Can you work these out from the model? Positions are in its coordinate system, mm. Face numbers are marked on the shaded views. A direction names the side the tool comes from. Give positions to 0.01 mm unless a question says otherwise; leave off trailing zeros. Order: outer loops, then holes, each group sorted by start corner. A loop starts at its lowest first (then second) coordinate and runs counter-clockwise, first axis right, second up. Notation, with made-up numbers: (-38, 87) - (8, 87) arc R32 ccw to (8, 123) - close; hole circle Ø8 at (58.25, 65). An arc over 180 degrees is marked (long way). One line per question, with ' | ' between items.
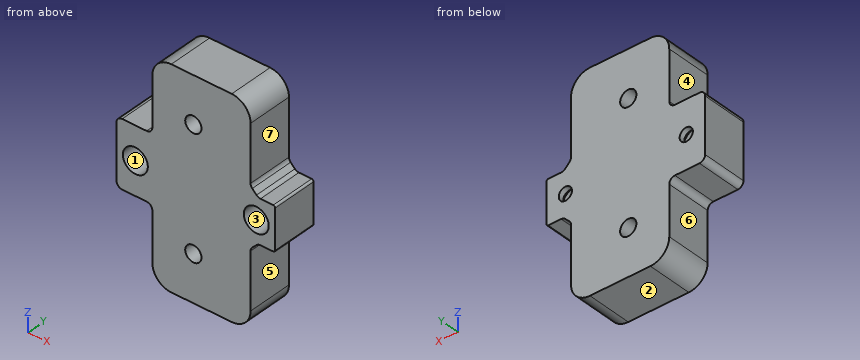
Autodesk Fusion 360 part; units mm, degrees
sketch "Sketch1" plane through (0, 0, 0) normal (0, 1, 0) x (1, 0, 0)
  line L0 (0, 0) -> (26, 0)
  line L1 (26, 0) -> (26, -56.5)
  line L2 (26, -56.5) -> (0, -56.5)
  line L3 (0, -56.5) -> (0, 0)
  line L4 (0, -37) -> (-9.5, -37)
  line L5 (-9.5, -37) -> (-9.5, -19.5)
  line L6 (-9.5, -19.5) -> (0, -19.5)
  line L7 (-9.5, -28.25) -> (0, -28.25) construction
  line L8 (26, -34) -> (32.5, -34)
  line L9 (32.5, -34) -> (32.5, -22.5)
  line L10 (32.5, -22.5) -> (26, -22.5)
  line L11 (26, -28.25) -> (32.5, -28.25) construction
  circle A0 centre (10.85, -44.25) radius 2.15
  circle A1 centre (10.85, -12.25) radius 2.15
  line L12 (10.85, -44.25) -> (10.85, -12.25) construction
  line L13 (0, -28.25) -> (10.85, -28.25) construction
  line L14 (8.7, -44.25) -> (10.85, -44.25) construction
  point P0 (8.7, -44.25)
  dimension "d2" = 26
  dimension "d3" = 56.5
  dimension "d4" = 9.5
  dimension "d5" = 17.5
  dimension "d6" = 6.5
  dimension "d7" = 11.5
  dimension "d8" = 32
  dimension "d9" = 4.3
  dimension "d10" = 8.7
extrude "Extrude1" add sketch "Sketch1" along normal blind 12
sketch "Sketch2" plane through (0, 0, 0) normal (0, -1, 0) x (1, 0, 0)
  circle A0 centre (10.85, 12.25) radius 2.15
  circle A1 centre (10.85, 44.25) radius 2.15
  line L0 (32.5, 34) -> (26, 34)
  line L1 (26, 34) -> (26, 56.5)
  line L2 (26, 56.5) -> (0, 56.5)
  line L3 (0, 56.5) -> (0, 37)
  line L4 (0, 37) -> (-9.5, 37)
  line L5 (-9.5, 37) -> (-9.5, 19.5)
  line L6 (-9.5, 19.5) -> (0, 19.5)
  line L7 (0, 19.5) -> (0, 0)
  line L8 (0, 0) -> (26, 0)
  line L9 (26, 0) -> (26, 22.5)
  line L10 (26, 22.5) -> (32.5, 22.5)
  line L11 (32.5, 22.5) -> (32.5, 34)
  line L12 (-9.5, 28.25) -> (32.5, 28.25) construction
  circle A2 centre (-4.5, 28.25) radius 3.3
  circle A3 centre (-4.5, 28.25) radius 1.75
  circle A4 centre (27.5, 28.25) radius 1.75
  circle A5 centre (27.5, 28.25) radius 3.3
  dimension "d20" = 3.5
  dimension "d21" = 6.6
  dimension "d22" = 5
  dimension "d23" = 5
extrude "Extrude2" cut sketch "Sketch2" against normal up to surface (12 mm away) contours A3 | A4
extrude "Extrude3" cut sketch "Sketch2" against normal up to surface (9 mm away) contours A2 | A5
chamfer "Chamfer2" distance 1.55 angle 45 2 edges at (-6.1316, 9, 27.6172) (25.8684, 9, 27.6172)
chamfer "Chamfer1" distance 2 angle 45 2 edges at (26, 6, 34) (26, 6, 22.5)
fillet "Fillet1" radius 1.5 8 edges at (0, 6, 37) (0, 6, 19.5) (26, 6, 36) (28, 6, 34) (26, 6, 20.5) (28, 6, 22.5) (-9.5, 6, 37) (-9.5, 6, 19.5)
fillet "Fillet2" radius 5 4 edges at (26, 6, 0) (0, 6, 56.5) (26, 6, 56.5) (0, 6, 0)
fillet "Fillet3" radius 0.5 2 edges at (32.5, 6, 34) (32.5, 6, 22.5)
equation "d11 = thickness"
equation "thickness = 12 mm"
(1) Will these pins go through, and if not, where does the flat tip stop? pin 1 (1 mm diameter, centred on x = 31, y = 7, fed in from -Z); pin 2 (7 mm diameter, centred on x = 10.85, z = 12.25, fed in from +Y); pin 3 (7 mm diameter, centred on x = -5.5, y = 5, fed in from +Z); pin 4 (5 mm diameter, centred on y = 8, z = 16.5, fed in from +X).
Answer below:
pin 1: z = 22.5 | pin 2: y = 12 | pin 3: z = 37 | pin 4: x = 26
(2) If we mould it in two halves opening along Z, with no side actions, what happens to the marked faces 1, 2, 3 and 4? For each: released by +Z, released by -Z, zero draft, split by the parting line, or undercut.
Answer below:
face 1: undercut | face 2: released by -Z | face 3: undercut | face 4: zero draft
(3) On a 3-axis mill with a long thin cutter (end or side, diameter ignored), from which of +Z, -Z, +X, -X, +Y, -Y can I reach the whole of each face in a straight line? I mean the marked faces 5, 6 and 7. Say none if no direction works.
Answer below:
face 5: -Z, +X, +Y, -Y | face 6: -Z, -X, +Y, -Y | face 7: +Z, +X, +Y, -Y
(4) Imagine slicing it at B-B (z = 44.25). List the corners of the cut face in (x, y) for me.
Answer below:
outline: (0, 0) - (8.7, 0) - (8.7, 12) - (0, 12) - close; (13, 0) - (26, 0) - (26, 12) - (13, 12) - close
(5) Imagine slicing it at D-D (y = 1). Count the separate pieces of the cut face and the enclosed holes in it, and give its area (3 significant figures).
Answer below:
separate pieces: 1 | enclosed holes: 4 | area: 1,600 mm^2
(6) Imagine slicing it at C-C (x = 10.85). List the corners of the cut face in (y, z) for me, and give its area (3 significant figures).
Answer below:
outline: (0, 0) - (12, 0) - (12, 10.1) - (0, 10.1) - close; (0, 14.4) - (12, 14.4) - (12, 42.1) - (0, 42.1) - close; (0, 46.4) - (12, 46.4) - (12, 56.5) - (0, 56.5) - close | area: 575 mm^2
(7) If I drill on line 1 (Z direction, x = -4.5, y = 6.75); line 2 (Z direction, x = 10.85, y = 2.5); line 3 (X direction, y = 4, z = 27), over which ranges is the centre line in solid material (lowest first)?
Answer below:
line 1: 19.5 to 24.95, 31.55 to 37 | line 2: 0 to 10.1, 14.4 to 42.1, 46.4 to 56.5 | line 3: -9.5 to -7.55, -1.45 to 24.45, 30.55 to 32.5
